Can you work these out from the model? Positions are in its coordinate system, mm. Face numbers are marked on the shaded views. A direction names the side the tool comes from. Round coordinates to 2 decimals unless told otherwise and drop trailing zeros. Order: outer loops, then holes, each group sorted by start corner. A loop starts at its lowest first (then second) coordinate and runs counter-clockwise, first axis right, second up. Notation, with made-up numbers: (-38, 43.25) - (-6, 43.25) arc R22 cw to (-6, 75.25) - close; hole circle Ø4 at (-39, -14.75). An arc over 180 degrees is marked (long way). Write item = value, one per line.
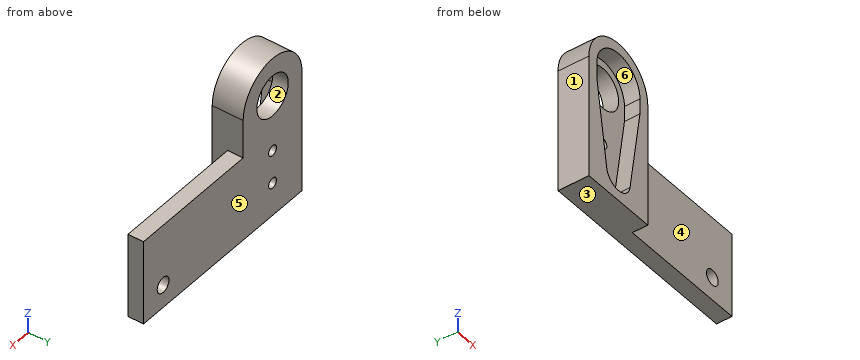
Autodesk Inventor part; units mm, degrees
ref_plane "YZ Plane" through (0, 0, 0) normal (1, 0, 0) x (0, 1, 0)
ref_plane "XZ Plane" through (0, 0, 0) normal (0, 1, 0) x (-1, 0, 0)
ref_plane "XY Plane" through (0, 0, 0) normal (0, 0, 1) x (1, 0, 0)
sketch "Sketch3" plane through (0, 0, 0) normal (0, 1, 0) x (-1, 0, 0)
  line L0 (0, 0) -> (0, -60)
  line L1 (0, 0) -> (60, 0) construction
  line L2 (0, -60) -> (12.519, -60)
  line L3 (0, 0) -> (25.4, 0)
  line L4 (25.4, 0) -> (25.4, 7.5)
  arc A0 (40.4, 7.5) -> (25.4, 7.5) centre (32.9, 7.5) ccw
  line L5 (40.4, 7.5) -> (40.4, -16.519)
  line L6 (40.4, -16.519) -> (12.519, -60)
  line L7 (0, -30) -> (5, -30)
  line L8 (5, -60) -> (5, -48)
  line L9 (5, 0) -> (5, -12)
  circle A1 centre (5, -12) radius 1.5
  circle A2 centre (5, -48) radius 1.5
  circle A3 centre (32.9, 7.5) radius 4
  line L10 (32.9, 7.5) -> (32.9, -3.512)
  line L11 (32.9, -3.512) -> (32.9, -10.02)
  circle A4 centre (32.9, -3.512) radius 1
  circle A5 centre (32.9, -10.02) radius 1
  dimension "d6" = 60
  dimension "d7" = 90
  dimension "d8" = 12.519
  dimension "d9" = 25.4
  dimension "d10" = 7.5
  dimension "d11" = 15
  dimension "d13" = 24.019
  dimension "d18" = 5
  dimension "d19" = 12
  dimension "d20" = 12
  dimension "d21" = 3
  dimension "d22" = 3
  dimension "d25" = 8
  dimension "d26" = 11.012
  dimension "d27" = 6.508
  dimension "d28" = 2
  dimension "d29" = 2
extrude "Extrusion1" add sketch "Sketch3" along normal blind 3
sketch "Sketch6" plane through (0, 3, 0) normal (0, 1, 0) x (1, 0, 0)
  circle A0 centre (-32.9, -7.5) radius 4
  circle A1 centre (-5, 48) radius 1.5
  circle A2 centre (-5, 12) radius 1.5
  circle A3 centre (-32.9, 10.02) radius 1
  circle A4 centre (-32.9, 3.512) radius 1
  line L0 (0, 0) -> (0, 60)
  line L1 (0, 60) -> (-12.519, 60)
  line L2 (-12.519, 60) -> (-40.4, 16.519)
  line L3 (-40.4, 16.519) -> (-40.4, -7.5)
  arc A5 (-40.4, -7.5) -> (-25.4, -7.5) centre (-32.9, -7.5) ccw
  line L4 (-25.4, -7.5) -> (-25.4, 0)
  line L5 (-25.4, 0) -> (0, 0)
  line L6 (-40.4, 16.519) -> (-25.4, 16.519)
  line L7 (-25.4, -7.5) -> (-25.4, 0)
  line L8 (-25.4, 16.519) -> (-25.4, 0)
  circle A6 centre (-32.9, -7.5) radius 5.5
  line L9 (-32.9, 10.02) -> (-32.9, 11.52)
  circle A7 centre (-32.9, 11.52) radius 3
  line L10 (-38.4, -7.5) -> (-38.4, -4.5)
  line L11 (-27.4, -7.5) -> (-27.4, -4.5)
  line L12 (-27.4, -4.5) -> (-29.9349, 11.9762)
  line L13 (-38.4, -4.5) -> (-35.8651, 11.9762)
  point P0 (0, 0)
  dimension "d31" = 11
  dimension "d32" = 1.5
  dimension "d33" = 6
  dimension "d34" = 3
extrude "Extrusion3" add sketch "Sketch6" against normal blind 6 contours L4 A5 L3 L6 L8
sketch "Sketch7" plane through (0, 3, 0) normal (0, 1, 0) x (1, 0, 0)
  line L0 (-40.4, 16.519) -> (-40.4, -7.5)
  line L1 (0, 60) -> (-12.519, 60)
  line L2 (0, 0) -> (0, 60)
  line L3 (-40.4, 60) -> (0, 60)
  line L4 (0, 60) -> (0, 16.519)
  line L5 (0, 16.519) -> (-40.4, 16.519)
  line L6 (-40.4, 16.519) -> (-40.4, 60)
extrude "Extrusion4" cut sketch "Sketch7" against normal blind 25.4
properties part number "exShort"
(1) Will these pins go through, and if not, where does the flat tip stop? P1, Ø1.5, axis at x = -22, z = -10, coming from the -Y side; P2, Ø1.8, axis at y = 0.5, z = 0, coming from the +X side; P3, Ø2.5, axis at y = -2, z = 6.5, coming from the +X side; P4, Ø3.5, axis at x = -10.5, y = 2, coming from the +Z side.
Computed:
P1 = 0
P2 = 0
P3 = -25.4
P4 = 0
(2) On a 3-axis mill with a long thin cutter (end or side, diameter ignored), from which of +Z, -Z, +X, -X, +Y, -Y can I reach the whole of each face in a straight line? I mean the marked faces 4, 5 and 6. Say none if no direction works.
Computed:
face_4 = +Z, -Z, +X, -Y
face_5 = +Z, -Z, +X, -X, +Y
face_6 = -Y
(3) Thinking about a two-plate mould opening in Z: for the marked faces 1, 2 and 3, which applies, +Z half, -Z half, draft (parallel to the pull), parting line (faces both ways), or undercut?
Computed:
face_1 = draft
face_2 = undercut
face_3 = -Z half
(4) If I drill on line 1 (Z direction, x = -32.9, y = 0.8); line 2 (X direction, y = 1.25, z = -10); line 3 (Z direction, x = -5, y = 1.7), over which ranges is the centre line in solid material (lowest first)? Write a range as from..to.
Computed:
line_1 = -16.52..-11.02, -9.02..-4.51, -2.51..3.5, 11.5..15
line_2 = -40.4..-33.9, -31.9..0
line_3 = -16.52..-13.5, -10.5..0
(5) If we section it at D-D (x = -6): Write out the boundary of the cut face in (y, z), plus the area to 3 significant figures.
Computed:
outline = (0, -16.52) - (3, -16.52) - (3, -13.12) - (0, -13.12) - close; (0, -10.88) - (3, -10.88) - (3, 0) - (0, 0) - close
area = 42.8 mm^2
(6) If we section it at B-B (z = 6): Write out the boundary of the cut face in (x, y).
Computed:
outline = (-40.4, -3) - (-38.4, -3) - (-38.4, 0) - (-36.61, 0) - (-36.61, 3) - (-40.4, 3) - close; (-29.19, 0) - (-27.4, 0) - (-27.4, -3) - (-25.4, -3) - (-25.4, 3) - (-29.19, 3) - close
(7) If we section it at A-A (x = -32.9): Write out the boundary of the cut face in (y, z).
Computed:
outline = (-3, -16.52) - (3, -16.52) - (3, -11.02) - (0, -11.02) - (0, -14.52) - (-3, -14.52) - close; (-3, 13) - (0, 13) - (0, 11.5) - (3, 11.5) - (3, 15) - (-3, 15) - close; (0, -9.02) - (3, -9.02) - (3, -4.51) - (0, -4.51) - close; (0, -2.51) - (3, -2.51) - (3, 3.5) - (0, 3.5) - close
(8) If we section it at C-C (y = 2.15): Write out the boundary of the cut face in (x, z).
Computed:
outline = (-40.4, -16.52) - (0, -16.52) - (0, 0) - (-25.4, 0) - (-25.4, 7.5) arc R7.5 ccw to (-40.4, 7.5) - close; hole circle Ø8 at (-32.9, 7.5); hole circle Ø2 at (-32.9, -10.02); hole circle Ø2 at (-32.9, -3.51); hole circle Ø3 at (-5, -12)
